Verification items for the finished model (mm, model axes). A direction names the side the tool comes from. Round coordinates to 2 decimals unless told otherwise and drop trailing zeros. Write each loop counter-clockwise with the first axis right and the second up, starting at its lowest first coordinate (ties: lowest second). Pieces come first, ordered by that corner, then holes.
from build123d import *

# Parameters (mm, degrees)
SKETCH_R      = 5.3
PAD_DEPTH     = 5
FILLET_R      = 10
FILLET001_R   = 1
SKETCH001_R   = 2
SKETCH001_W   = 9.475223
SKETCH001_H   = 23.68809
SKETCH001_W_2 = 11
SKETCH001_W_3 = 4.903309
SKETCH001_H_2 = 2.2
POCKET_DEPTH  = 5
SKETCH002_W   = 8
SKETCH002_H   = 4
PAD001_DEPTH  = 5
FILLET002_R   = 1.5


with BuildPart() as part:
    # Sketch → Pad (new body)
    with BuildSketch(Plane.XY):
        Polygon((30.887989, 10.25), (30.887989, 16.25), (-39.112011, 16.25), (-39.112011, -16.25), (30.887989, -16.25), (30.887989, -10.25), (10.887989, -10.25), (10.887989, 10.25), align=None)
        with Locations((-16.112011, 0)):
            Circle(SKETCH_R, mode=Mode.SUBTRACT)
    extrude(amount=PAD_DEPTH)

    # Fillet
    fillet_edges = [part.edges().sort_by_distance(p)[0] for p in [
        (-39.112011, -16.25, 2.5),
        (-39.112011, 16.25, 2.5),
    ]]
    fillet(fillet_edges, radius=FILLET_R)

    # Fillet001
    fillet001_edges = [part.edges().sort_by_distance(p)[0] for p in [
        (30.887989, -16.25, 2.5),
        (30.887989, 16.25, 2.5),
    ]]
    fillet(fillet001_edges, radius=FILLET001_R)

    # Sketch001 (on Face5 of Fillet001) → Pocket (cut)
    with BuildSketch(Plane.XY.offset(5)):
        with Locations((6.887989, 6.25)):
            Circle(SKETCH001_R)
        with Locations((6.887989, -6.25)):
            Circle(SKETCH001_R)
        with Locations((-28.9485835, 0)):
            Rectangle(SKETCH001_W, SKETCH001_H)
        with Locations((-2.4204911845, 0)):
            Rectangle(SKETCH001_W_2, SKETCH001_H)
        with Locations((8.4363345, 0)):
            Rectangle(SKETCH001_W_3, SKETCH001_H_2)
    extrude(amount=-POCKET_DEPTH, mode=Mode.SUBTRACT)

    # Sketch002 (on Face5 of Pocket) → Pad001 (join)
    with BuildSketch(Plane.XY.offset(5)):
        with Locations((-16.112011, 9.067142847)):
            Rectangle(SKETCH002_W, SKETCH002_H)
        with Locations((-16.112011, -9.067142847)):
            Rectangle(SKETCH002_W, SKETCH002_H)
    extrude(amount=PAD001_DEPTH)

    # Fillet002
    fillet002_edges = [part.edges().sort_by_distance(p)[0] for p in [
        (-16.112011, 11.067143, 10),
        (-12.112011, 9.067143, 10),
        (-16.112011, 7.067143, 10),
        (-20.112011, 9.067143, 10),
        (-16.112011, -7.067143, 10),
        (-12.112011, -9.067143, 10),
        (-16.112011, -11.067143, 10),
        (-20.112011, -9.067143, 10),
    ]]
    fillet(fillet002_edges, radius=FILLET002_R)


solid = part.part
Q1. Sectioned sample at B-B (x = 26.5). Enter the section's corners in (y, z), plus the area to 3 significant figures.
Recorded:
outline: (-16.25, 0) - (-10.25, 0) - (-10.25, 5) - (-16.25, 5) - close; (10.25, 0) - (16.25, 0) - (16.25, 5) - (10.25, 5) - close
area: 60.0 mm2
Q2. Sectioned sample at A-A (y = 0). Enter the section's corners in (x, z), plus the area to 3 significant figures.
Recorded:
outline: (-39.11, 0) - (-33.69, 0) - (-33.69, 5) - (-39.11, 5) - close; (-24.21, 0) - (-21.41, 0) - (-21.41, 5) - (-24.21, 5) - close; (-10.81, 0) - (-7.92, 0) - (-7.92, 5) - (-10.81, 5) - close; (3.08, 0) - (5.98, 0) - (5.98, 5) - (3.08, 5) - close
area: 70.1 mm2
Q3. Sectioned sample at C-C (z = 3). Enter the section's corners in (x, y).
Recorded:
outline: (-39.11, -6.25) arc R10 ccw to (-29.11, -16.25) - (29.89, -16.25) arc R1 ccw to (30.89, -15.25) - (30.89, -10.25) - (10.89, -10.25) - (10.89, -1.1) - (5.98, -1.1) - (5.98, 1.1) - (10.89, 1.1) - (10.89, 10.25) - (30.89, 10.25) - (30.89, 15.25) arc R1 ccw to (29.89, 16.25) - (-29.11, 16.25) arc R10 ccw to (-39.11, 6.25) - close; hole (-33.69, -11.84) - (-24.21, -11.84) - (-24.21, 11.84) - (-33.69, 11.84) - close; hole circle Ø10.6 at (-16.11, 0); hole (-7.92, -11.84) - (3.08, -11.84) - (3.08, 11.84) - (-7.92, 11.84) - close; hole circle Ø4 at (6.89, -6.25); hole circle Ø4 at (6.89, 6.25)
Q4. Depth check by flat-ended pin: P1, Ø4, axis at y = 6.5, z = 1.5, coming from the +X side; P2, Ø3, axis at x = -17, z = 7.5, coming from the -Y side; P3, Ø2, axis at x = -14.5, z = 8.5, coming from the +Y side; P4, Ø3, axis at x = 6.89, y = -6.25, coming from the -Z side. Enter the tip coordinate at first touch or a pass-through.
Recorded:
P1: stops at x = 10.89
P2: stops at y = -11.07
P3: stops at y = 11.07
P4: passes through
Q5. Sectioned sample at D-D (z = 7.75). Enter the section's corners in (x, y), plus the area to 3 significant figures.
Recorded:
outline: (-20.11, -11.07) - (-12.11, -11.07) - (-12.11, -7.07) - (-20.11, -7.07) - close; (-20.11, 7.07) - (-12.11, 7.07) - (-12.11, 11.07) - (-20.11, 11.07) - close
area: 64.0 mm2
Q6. Tool access check on faces 1 (the flat face through (21, 10.25, 2)), 2 (the flat face through (-16, -7.067, 7)), 3 (the flat face through (-20.112, -9, 7)), 4 (the flat face through (-24.211, 0, 3)), 5 (the flat face through (-12.112, -9, 7)). Record the directions out of +Z, -Z, +X, -X, +Y, -Y that give a thin tool (end or side, any length) a straight path to the whole face; none if there is none.
Recorded:
face 1: +Z, -Z, +X
face 2: +Z, +X, -X
face 3: +Z, -X, +Y, -Y
face 4: +Z, -Z
face 5: +Z, +X, +Y, -Y
Q7. Material ranges on line 1 along X through (y, z) = (-2.5, 0.75); line 2 along Y through (x, z) = (14.5, 3.25); line 3 along X through (y, z) = (1, 2.5), recorded low to high.
Recorded:
line 1: x = -39.11 to -33.69, -24.21 to -20.79, -11.44 to -7.92, 3.08 to 10.89
line 2: y = -16.25 to -10.25, 10.25 to 16.25
line 3: x = -39.11 to -33.69, -24.21 to -21.32, -10.91 to -7.92, 3.08 to 5.98
Q8. Release check for a two-part mould opening along Y. For faces 6 (the flat face through (-12, 4, 0)), 7 (the cylindrical face through (-36.105, 13.398, 2.535)), 8 (the flat face through (-16, -11.067, 7)), 9 (the flat face through (21, -10.25, 2)) record: released by +Y, released by -Y, zero draft, split by the parting line, or undercut.
Recorded:
face 6: zero draft
face 7: released by +Y
face 8: released by -Y
face 9: undercut
